Source: CAD feature listing. Evaluate the final solid. Frame: model axes, mm. A direction names the side the tool comes from. Coordinates: 2 decimals unless noted, no trailing zeros. Write each loop counter-clockwise with the first axis right and the second up, starting at its lowest first coordinate (ties: lowest second). Pieces come first, ordered by that corner, then holes. Notation, with made-up numbers: (-17, -29) - (19, -29) arc R25 ccw to (19, 9) - close; hole circle Ø5 at (49, 2.25). An arc over 180 degrees is marked (long way). One line per question, with ' | ' between items. Start each with the question number.
Q1. Access query for faces 4 (the face through (25.12, 273.25, -19.06)), 5 (the face through (25, 309, -50.8)), 6 (the face through (25, 606.425, -26)). Directions: +Z, -Z, +X, -X, +Y, -Y. A direction counts if a zero-diameter tool reaches every point of the face in a straight line with its end or side. Return the directions, or none.
Q2. Cut plane A-A, the plane y = 315.5. Return loops of the section in (x, z).
Q3. Line query: line 1 (Z direction, x = 21, y = 413); line 2 (Y direction, x = 17, z = -35) (3 decimals); line 3 (X direction, y = 31, z = -28). Output: solid intervals per line, ascending.
Q4. Contact query for flat-ended pins moving along their axis: P1, Ø6.5, axis at x = 25.5, z = -26, coming from the -Y side; P2, Ø7.5, axis at x = 25.4, z = -25.4, coming from the +Y side (3 decimals). Output: stop coordinate, or through.
Q5. Draft query along Y for faces 1 (the face through (0, 301, -25)), 2 (the face through (37.84, 528.1, -10.6)), 3 (the face through (8, 609.6, -25)). Return one class per face: +Y half, -Y half, draft (parallel to the pull), parting line (faces both ways), or undercut.
Autodesk Inventor part; units mm, degrees
ref_plane "Work Plane2" through (50.8, 0, 0) normal (0.7071, 0, 0.7071) x (0, -1, 0)
ref_plane "YZ Plane" through (0, 0, 0) normal (1, 0, 0) x (0, 1, 0)
ref_plane "XZ Plane" through (0, 0, 0) normal (0, 1, 0) x (-1, 0, 0)
sketch "Sketch1" plane through (0, 0, 0) normal (1, 0, 0) x (0, 1, 0)
  line L0 (0, 0) -> (609.6, 0)
  line L1 (609.6, 0) -> (609.6, -50.8)
  line L2 (609.6, -50.8) -> (0, -50.8)
  line L3 (0, -50.8) -> (0, 0)
  dimension "d0" = 609.6
  dimension "d1" = 50.8
extrude "Extrusion1" add sketch "Sketch1" along normal blind 50.8
ref_plane "Work Plane2" through (50.8, 0, 0) normal (0.7071, 0, 0.7071) x (0, -1, 0)
sketch "Sketch4" plane through (50.8, 0, 0) normal (0.7071, 0, 0.7071) x (0, -1, 0)
  line L0 (-609.6, 0) -> (-533.4, 0)
  line L1 (0, 0) -> (-3.175, 0)
  point P0 (0, -35.921)
  dimension "d8" = 76.2
  dimension "d16" = 3.175
hole "Hole1" at (50.8, 533.4, 0) direction (-0.7071, 0, -0.7071) diameter 11.1125 depth 35.9156
sketch "Sketch6" plane through (50.8, 0, 0) normal (0.7071, 0, 0.7071) x (0, -1, 0)
  line L0 (0, -35.921) -> (0, 0)
  line L1 (0, 0) -> (-3.175, 0)
  line L2 (-609.6, 0) -> (0, 0)
  dimension "d17" = 3.175
hole "Hole2" at (50.8, 3.175, 0) direction (-0.7071, 0, -0.7071) diameter 12.7 depth 42.2656
sketch "Sketch10" plane through (0, 0, -50.8) normal (0, -1, 0) x (1, 0, 0)
  line L0 (0, 0) -> (25.3962, 25.3962)
  line L1 (0, 0) -> (50.8, 0)
  point P0 (0, 50.8)
  point P1 (50.8, 50.8)
  dimension "d34" = 35.9156
  dimension "d35" = 45
hole "Hole4" at (25.3962, 0, -25.4038) direction (0, 1, 0) diameter 12.7 depth 538.9626
sketch "Sketch11" plane through (0, 609.6, 0) normal (0, 1, 0) x (1, 0, 0)
  line L0 (12.7, 38.1) -> (38.1, 38.1)
  line L1 (38.1, 38.1) -> (38.1, 12.7)
  line L2 (38.1, 12.7) -> (12.7, 12.7)
  line L3 (12.7, 12.7) -> (12.7, 38.1)
  line L4 (0, 50.8) -> (0, 0)
  line L5 (0, 50.8) -> (50.8, 50.8)
  dimension "d43" = 25.4
  dimension "d44" = 25.4
  dimension "d45" = 12.7
  dimension "d46" = 12.7
extrude "Extrusion2" cut sketch "Sketch11" against normal blind 3.175
properties part number "LegOutlet" material "Wood (Birch)"
Reply:
1) face 4: -Y | face 5: -Z, +X, -X, +Y, -Y | face 6: +Y
2) outline: (0, -50.8) - (50.8, -50.8) - (50.8, 0) - (0, 0) - close; hole circle Ø12.7 at (25.4, -25.4)
3) line 1: z = -50.8 to -29.99, -20.82 to 0 | line 2: y = 0 to 606.425 | line 3: x = 0 to 19.6, 31.19 to 50.8
4) P1: stops at y = 538.96 | P2: stops at y = 606.425
5) face 1: draft | face 2: undercut | face 3: +Y half
